```python
from build123d import *

# Parameters (mm, degrees)
SKETCH1_W             = 25
SKETCH1_H             = 50
BOSS_EXTRUDE1_DEPTH   = 30.875
CUT_EXTRUDE1_REACH    = 82.432
M6_TAPPED_HOLE1_D     = 5
M6_TAPPED_HOLE1_DEPTH = 17
M6_TAPPED_HOLE1_TIP   = 1.502151548


with BuildPart() as part:
    # Sketch1 → Boss-Extrude1 (new, symmetric)
    with BuildSketch(Plane.XY):
        with Locations((0, -25)):
            Rectangle(SKETCH1_W, SKETCH1_H)
    extrude(amount=BOSS_EXTRUDE1_DEPTH, both=True)

    # Sketch2 → Cut-Extrude1 (cut, up to next)
    with BuildSketch(Plane(origin=(0, 0, -30.875), x_dir=(-1, 0, 0), z_dir=(0, 0, -1)), mode=Mode.PRIVATE) as cut_extrude1_sk1:
        with BuildLine():
            Line((-2.363703305, -46.96472382), (-3.177003107, -50))
            Line((-3.177003107, -50), (6.177003107, -50))
            Line((6.177003107, -50), (5.363703305, -46.96472382))
            ThreePointArc((5.363703305, -46.96472382), (1.5, -44), (-2.363703305, -46.96472382))
        make_face()
    cut_extrude1_tool1 = extrude(cut_extrude1_sk1.sketch, amount=-CUT_EXTRUDE1_REACH, mode=Mode.PRIVATE) & part.part
    add(cut_extrude1_tool1.solids().sort_by_distance((-1.5, -47.423831, -30.875))[0], mode=Mode.SUBTRACT)

    # M6 Tapped Hole1
    with Locations(Plane(origin=(0, 0, 0), x_dir=(1, 0, 0), z_dir=(0, 1, 0))):
        with Locations((0, 21), (0, -21)):
            Hole(M6_TAPPED_HOLE1_D / 2, depth=M6_TAPPED_HOLE1_DEPTH)
            with Locations((0, 0, -(M6_TAPPED_HOLE1_DEPTH + M6_TAPPED_HOLE1_TIP / 2))):  # 118° drill point
                Cone(0, M6_TAPPED_HOLE1_D / 2, M6_TAPPED_HOLE1_TIP, mode=Mode.SUBTRACT)


solid = part.part
```
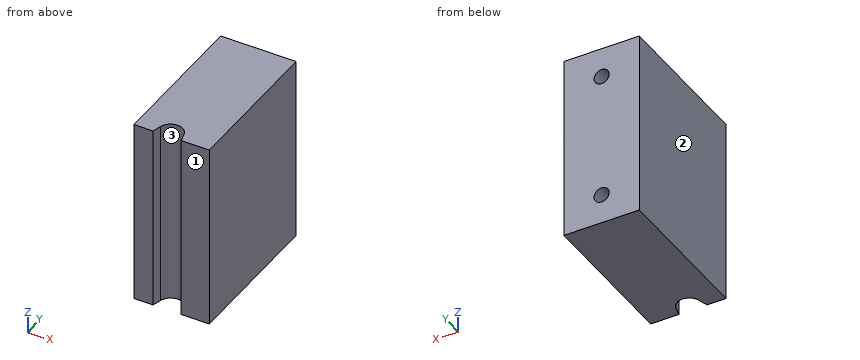
The model under review builds one solid part; all positions refer to its coordinate system, in mm. Face numbers are marked on the shaded views. Round coordinates to 2 decimals unless told otherwise and drop trailing zeros. Loops run counter-clockwise (first coordinate to the right, second up) from the corner with the lowest first, then second, coordinate; pieces in that order, holes last. Notation, with made-up numbers: (76, 17.5) - (81, 17.5) arc R20 ccw to (81, 40.5) - close; hole circle Ø5 at (-15.75, -19.75). An arc over 180 degrees is marked (long way). Write each question's results on one line, items separated by ' | '. Start each with the question number.
Q1. Take a section at C-C on y = -45.5. Give the boundary of the cut face in (x, z) (1 decimal).
Q2. Take a section at B-B on z = -12.5. Give the boundary of the cut face in (x, y).
Q3. Take a section at A-A on y = -7. Give the boundary of the cut face in (x, z) (3 decimals).
Q4. Draft analysis for pull direction X (two halves, no side actions). For the marked faces 1, 2 and 3, state which applies: pulls with the +X half, pulls with the -X half, needs draft (parallel to the pull), parting line crosses it, or undercut.
Q5. Wall thickness on line 1 along Z through (x, y) = (0, -10.5) (3 decimals); line 2 along X through (y, z) = (-4.5, -21); line 3 along Z through (x, y) = (1, -2) (3 decimals): over which ranges is each line inside the solid? List them lowest first. Write a range as [from, to].
Data:
1) outline: (-12.5, -30.9) - (-4.6, -30.9) - (-4.6, 30.9) - (-12.5, 30.9) - close; (1.6, -30.9) - (12.5, -30.9) - (12.5, 30.9) - (1.6, 30.9) - close
2) outline: (-12.5, -50) - (-6.18, -50) - (-5.36, -46.96) arc R4 cw to (2.36, -46.96) - (3.18, -50) - (12.5, -50) - (12.5, 0) - (-12.5, 0) - close
3) outline: (-12.5, -30.875) - (12.5, -30.875) - (12.5, 30.875) - (-12.5, 30.875) - close; hole circle Ø5 at (0, -21); hole circle Ø5 at (0, 21)
4) face 1: needs draft | face 2: pulls with the -X half | face 3: undercut
5) line 1: z = [-30.875, -23.5], [-18.5, 18.5], [23.5, 30.875] | line 2: x = [-12.5, -2.5], [2.5, 12.5] | line 3: z = [-30.875, -23.291], [-18.709, 18.709], [23.291, 30.875]
